Here's how the part is built. I have some questions about the finished solid (model axes, mm). Give positions to 0.01 mm unless a question says otherwise; leave off trailing zeros. Order: outer loops, then holes, each group sorted by start corner. A loop starts at its lowest first (then second) coordinate and runs counter-clockwise, first axis right, second up.
Autodesk Inventor part; units mm, degrees
ref_plane "YZ Plane" through (0, 0, 0) normal (1, 0, 0) x (0, 1, 0)
ref_plane "XZ Plane" through (0, 0, 0) normal (0, 1, 0) x (-1, 0, 0)
ref_plane "XY Plane" through (0, 0, 0) normal (0, 0, 1) x (1, 0, 0)
sketch "Sketch1" plane through (0, 0, 0) normal (1, 0, 0) x (0, 1, 0)
  line L0 (-69.85, 342.9) -> (-69.85, -342.9)
  line L1 (-69.85, -342.9) -> (69.85, -342.9)
  line L2 (69.85, -342.9) -> (69.85, 342.9)
  line L3 (69.85, 342.9) -> (-69.85, 342.9)
  line L4 (-69.85, 342.9) -> (69.85, -342.9) construction
  line L5 (-69.85, -342.9) -> (69.85, 342.9) construction
  point P0 (0, 0)
  dimension "width" = 685.8
  dimension "height" = 139.7
extrude "Extrusion1" add sketch "Sketch1" along normal blind 6.35
sketch "Sketch2" plane through (6.35, 0, 0) normal (1, 0, 0) x (0, 0, -1)
  line L0 (-317.5, 38.1) -> (-63.5, 38.1) construction
  line L1 (-317.5, 28.575) -> (-63.5, 28.575)
  line L2 (-63.5, 47.625) -> (-317.5, 47.625)
  arc A0 (-317.5, 47.625) -> (-317.5, 28.575) centre (-317.5, 38.1) ccw
  arc A1 (-63.5, 28.575) -> (-63.5, 47.625) centre (-63.5, 38.1) ccw
  line L3 (342.9, 69.85) -> (-342.9, 69.85)
  line L4 (-342.9, 69.85) -> (-342.9, -69.85)
  line L5 (63.5, -38.1) -> (317.5, -38.1) construction
  line L6 (63.5, -47.625) -> (317.5, -47.625)
  line L7 (317.5, -28.575) -> (63.5, -28.575)
  arc A2 (63.5, -28.575) -> (63.5, -47.625) centre (63.5, -38.1) ccw
  arc A3 (317.5, -47.625) -> (317.5, -28.575) centre (317.5, -38.1) ccw
  line L8 (-342.9, -69.85) -> (342.9, -69.85)
  line L9 (342.9, -69.85) -> (342.9, 69.85)
  point P0 (0, 0)
  point P1 (-190.5, 38.1)
  point P2 (190.5, -38.1)
  dimension "slot_center_from_top" = 31.75
  dimension "slot_center_from_side" = 152.4
  dimension "slot_radius" = 9.525
  dimension "d7" = 31.75
  dimension "d8" = 152.4
  dimension "d9" = 9.525
  dimension "length_of_slot" = 254
  dimension "d13" = 254
extrude "Extrusion2" cut sketch "Sketch2" against normal through all contours A0 L2 A1 L1 | A2 L7 A3 L6
sketch "Sketch3" plane through (0, 0, 0) normal (-1, 0, 0) x (0, 0, 1)
  line L0 (-342.9, 69.85) -> (342.9, 69.85) construction
  line L1 (6.3584, 69.85) -> (6.3584, -72.7678) construction
  line L2 (342.9, 69.85) -> (342.9, -69.85) construction
  line L3 (-6.3584, 69.85) -> (-6.3584, -69.85) construction
  line L4 (-342.9, -69.85) -> (-342.9, 69.85) construction
  line L5 (-6.3584, 61.976) -> (6.3584, 61.976) construction
  line L6 (-6.3584, -61.976) -> (6.3584, -61.976) construction
  line L7 (342.9, -69.85) -> (-342.9, -69.85) construction
  line L8 (-6.3584, 14.224) -> (6.3584, 14.224) construction
  line L9 (-6.3584, -14.224) -> (6.3584, -14.224) construction
  point P0 (0, 0)
  point P1 (80.6051, 237.827)
  point P2 (47.886, -92.9067)
  dimension "Vertical_Line_For_Bolt_Holes" = 336.5416
  dimension "d15" = 336.5416
  dimension "First_Horizontal_Line" = 7.874
  dimension "d17" = 7.874
  dimension "Second_Horizontal_Line" = 47.752
  dimension "d19" = 47.752
hole "Hole1" at (0, 61.976, 6.3584) at (0, -61.976, -6.3584) at (0, 237.827, 80.6051) at (0, -92.9067, 47.886) at (0, 14.224, 6.3584) at (0, -14.224, -6.3584) direction (1, 0, 0) diameter 6.35 end through all
equation "\"d9\" = slot_radius"
equation "\"d13\" = length_of_slot"
equation "\"d15\" = Vertical_Line_For_Bolt_Holes"
equation "\"d17\" = First_Horizontal_Line"
properties part number "Plot for Gripper-09" material "Aluminum 6061"
Q1. If we section it at B-B on y = -38.1: List the corners of the cut face in (x, z) for me (3 decimals), plus the area to 3 significant figures.
Filled sheet:
outline: (0, -342.9) - (6.35, -342.9) - (6.35, -327.025) - (0, -327.025) - close; (0, -53.975) - (6.35, -53.975) - (6.35, 342.9) - (0, 342.9) - close
area: 2,620 mm2
Q2. If we section it at A-A on z = -252.5: List the corners of the cut face in (x, y) for me (3 decimals).
Filled sheet:
outline: (0, -69.85) - (6.35, -69.85) - (6.35, -47.625) - (0, -47.625) - close; (0, -28.575) - (6.35, -28.575) - (6.35, 69.85) - (0, 69.85) - close
Q3. I'm going to push a flat-ended pin straight in: P1, Ø4, axis at y = -13, z = 250, coming from the -X side. Where does the tip first touch, or does it pass through?
Filled sheet:
P1: stops at x = 0
Q4. If we section it at C-C on x = 1.25: List the corners of the cut face in (y, z) for me (3 decimals), plus the area to 3 significant figures.
Filled sheet:
outline: (-69.85, -342.9) - (69.85, -342.9) - (69.85, 342.9) - (-69.85, 342.9) - close; hole circle Ø6.35 at (-61.976, -6.358); hole (-47.625, -317.5) arc R9.525 ccw to (-28.575, -317.5) - (-28.575, -63.5) arc R9.525 ccw to (-47.625, -63.5) - close; hole circle Ø6.35 at (-14.224, -6.358); hole circle Ø6.35 at (14.224, 6.358); hole (28.575, 63.5) arc R9.525 ccw to (47.625, 63.5) - (47.625, 317.5) arc R9.525 ccw to (28.575, 317.5) - close; hole circle Ø6.35 at (61.976, 6.358)
area: 85,400 mm2
Q5. I need wall thicknesses on L1, parallel to Y at x = 0.75, z = 144.5 (3 decimals); L2, parallel to Y at x = 5, z = -249.5 (3 decimals); L3, parallel to Z at x = 1.5, y = 37.5. Which ranges of each line are inside material? Lowest first, please.
Filled sheet:
L1: y = -69.85 to 28.575, 47.625 to 69.85
L2: y = -69.85 to -47.625, -28.575 to 69.85
L3: z = -342.9 to 53.99, 327.01 to 342.9
